Could you check a few things on this drawing? It's one solid part, dimensions in mm from its lowest x, y, z. Round coordinates to 2 decimals unless told otherwise and drop trailing zeros. Loops run counter-clockwise (first coordinate to the right, second up) from the corner with the lowest first, then second, coordinate; pieces in that order, holes last. Notation, with made-up numbers: M -19,64 L 34,64 A20 cw 34,77 Z; hole C -2,62.5 d7. An arc over 180 degrees is marked long. Answer as CSV lines item,"result".
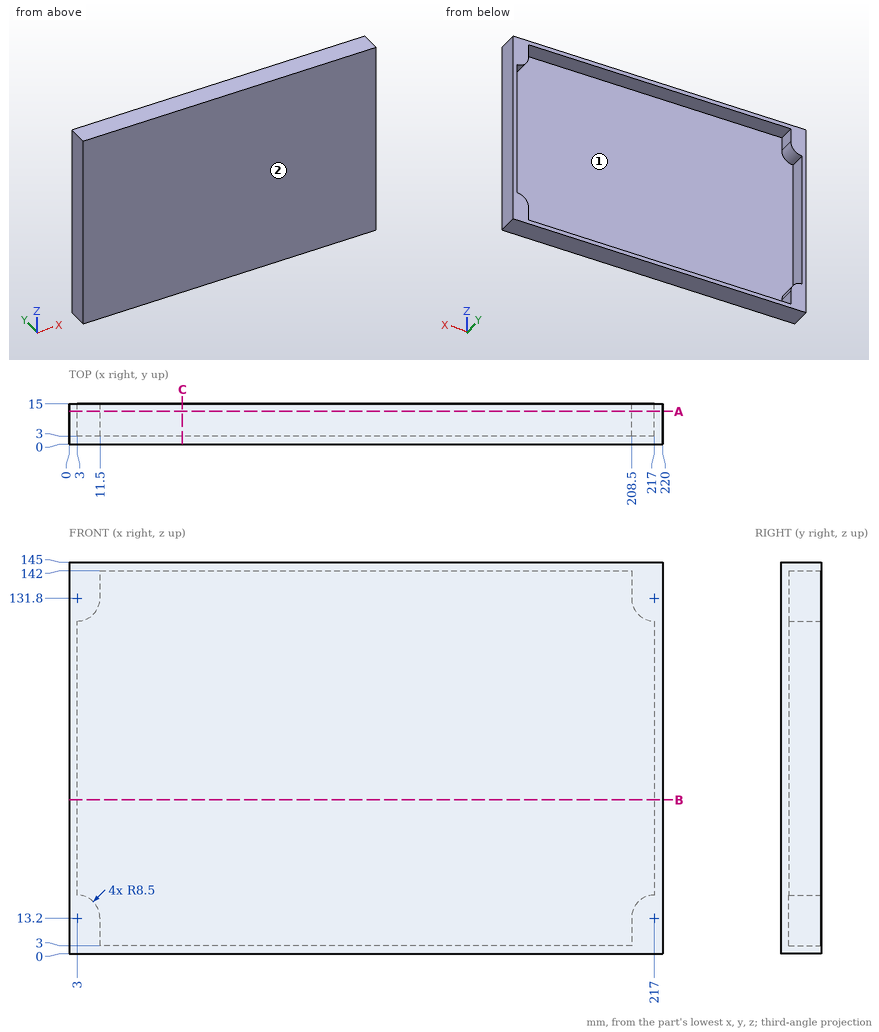
Item 1: If we section it at B-B on z = 57: Write out the boundary of the cut face in (x, y), then the cut area to 3 significant figures.
Output:
outline,"M 0,0 L 220,0 L 220,15 L 217,15 L 217,3 L 3,3 L 3,15 L 0,15 Z"
area,"732 mm2"
Item 2: If we section it at C-C on x = 42: Write out the boundary of the cut face in (y, z).
Output:
outline,"M 0,0 L 15,0 L 15,3 L 3,3 L 3,142 L 15,142 L 15,145 L 0,145 Z"
Item 3: We'd pull the mould along Z, two halves only. Please class the marked faces 1 and 2: released by +Z, released by -Z, zero draft, split by the parting line, or undercut.
Output:
face 1,"undercut"
face 2,"zero draft"
Item 4: If we section it at A-A on y = 12.25: Write out the boundary of the cut face in (x, z), then the cut area to 3 significant figures.
Output:
outline,"M 0,0 L 220,0 L 220,145 L 0,145 Z; hole M 3,21.7 A8.5 cw 11.5,13.2 L 11.5,3 L 208.5,3 L 208.5,13.2 A8.5 cw 217,21.7 L 217,123.3 A8.5 cw 208.5,131.8 L 208.5,142 L 11.5,142 L 11.5,131.8 A8.5 cw 3,123.3 Z"
area,"2,730 mm2"
Item 5: If I drill on line 1 along X through (y, z) = (12.25, 93.5); line 2 along Z through (x, y) = (103, 6.75); line 3 along X through (y, z) = (5.75, 10.5), over which ranges is the centre line in solid material (lowest first)? Write a range as from..to.
Output:
line 1,"x = 0..3, 217..220"
line 2,"z = 0..3, 142..145"
line 3,"x = 0..11.5, 208.5..220"
Item 6: Will this pin go through, and if not, where does the flat tip stop? pin 1 (4 mm diameter, centred on x = 162.5, z = 120, fed in from +Y).
Output:
pin 1,"stops at y = 3"
